Autodesk Inventor part; units mm, degrees
ref_plane "YZ Plane" through (0, 0, 0) normal (1, 0, 0) x (0, 1, 0)
ref_plane "XZ Plane" through (0, 0, 0) normal (0, 1, 0) x (-1, 0, 0)
ref_plane "XY Plane" through (0, 0, 0) normal (0, 0, 1) x (1, 0, 0)
sketch "Sketch1" plane through (0, 0, 0) normal (0, 1, 0) x (-1, 0, 0)
  line L0 (0, 0) -> (230, 0)
  line L1 (230, 0) -> (230, -230)
  line L2 (230, -230) -> (0, -230)
  line L3 (0, -230) -> (0, 0)
  dimension "d0" = 230
  dimension "d1" = 230
extrude "Extrusion1" add sketch "Sketch1" along normal blind 4
chamfer "Chamfer1" distance 2 angle 45 4 edges at (-230, 2, 0) (-230, 2, -230) (0, 2, -230) (0, 2, 0)
sketch "Sketch5" plane through (0, 4, 0) normal (0, 1, 0) x (1, 0, 0)
  line L0 (-215, 215) -> (-15, 215)
  line L1 (-15, 215) -> (-15, 15)
  line L2 (-15, 15) -> (-215, 15)
  line L3 (-215, 15) -> (-215, 215)
  point P0 (0, 0)
  dimension "d29" = 200
  dimension "d30" = 200
  dimension "d31" = 15
  dimension "d32" = 15
extrude "Extrusion5" cut sketch "Sketch5" against normal through all
properties part number "MouldBase20"
The model under review builds one solid part; all positions refer to its coordinate system, in mm. Round coordinates to 2 decimals unless told otherwise and drop trailing zeros. Order: outer loops, then holes, each group sorted by start corner. A loop starts at its lowest first (then second) coordinate and runs counter-clockwise, first axis right, second up. Notation, with made-up numbers: (-27.75, -29) - (-3.75, -29) arc R13 ccw to (-3.75, -8) - close; hole circle Ø6 at (27.5, 54). An arc over 180 degrees is marked (long way). Answer in a Markdown table with one row per item.
(1) Take a section at B-B on x = -173.5. Write out the cut boundary in (y, z).
Result set:
| item | result |
|---|---|
| outline | (0, -230) - (4, -230) - (4, -215) - (0, -215) - close; (0, -15) - (4, -15) - (4, 0) - (0, 0) - close |
(2) Take a section at C-C on y = 3.4. Write out the cut boundary in (x, z), plus the area to 3 significant figures.
Result set:
| item | result |
|---|---|
| outline | (-230, -228) - (-228, -230) - (-2, -230) - (0, -228) - (0, -2) - (-2, 0) - (-228, 0) - (-230, -2) - close; hole (-215, -215) - (-15, -215) - (-15, -15) - (-215, -15) - close |
| area | 12,900 mm2 |
(3) For line 1 (Z direction, x = -181.5, y = 2.1), list the stretches that pass through material, from the lowest coordinate up. Write a range as from..to.
Result set:
| item | result |
|---|---|
| line 1 | z = -230..-215, -15..0 |
(4) Take a section at A-A on z = -91.5. Write out the cut boundary in (x, y).
Result set:
| item | result |
|---|---|
| outline | (-230, 0) - (-215, 0) - (-215, 4) - (-230, 4) - close; (-15, 0) - (0, 0) - (0, 4) - (-15, 4) - close |
